Drawing for the job (mm, zero at the part's lowest x, y, z). A direction names the side the tool comes from. Round coordinates to 2 decimals unless told otherwise and drop trailing zeros. Write each loop counter-clockwise with the first axis right and the second up, starting at its lowest first coordinate (ties: lowest second). Pieces come first, ordered by that corner, then holes.
Item 1: Band-saw the part on D-D, the plane z = 5.5. Write the cut outline in (x, y), then the cut area to 3 significant figures.
Item 2: Mould opens along Z. For the marked faces 3, 4, 5 and 6 say: +Z half, -Z half, draft (parallel to the pull), parting line (faces both ways), or undercut.
Item 3: Band-saw the part on A-A, the plane y = 7.5. Write the cut outline in (x, z).
Item 4: Wall check: probe 1 along Y at (x, z) = (7.5, 4.5); probe 2 along Z at (x, y) = (4.5, 13.75); probe 3 along X at (y, z) = (6.25, 10) (1 decimal). Give the ranges that are in metal, low to high.
Item 5: 3-axis set-ups, long thin cutter, end or side, ignore diameter. For the marked faces 1 and 2: which of +Z, -Z, +X, -X, +Y, -Y reach the whole face in a straight line?
Item 6: Drop flat-ended pins along their axis: pin 1 Ø4 at (x, z) = (10, 6.5) entering from -Y; pin 2 Ø7.5 at (x, y) = (4.5, 6.5) entering from -Z; pin 3 Ø6 at (x, z) = (13, 4) entering from -Y (1 decimal); pin 4 Ø4.5 at (x, y) = (7.5, 7.5) entering from +Z. Give the stop position or say it passes through.
Item 7: Band-saw the part on C-C, the plane y = 12.25. Write the cut outline in (x, z), then the cut area to 3 significant figures.
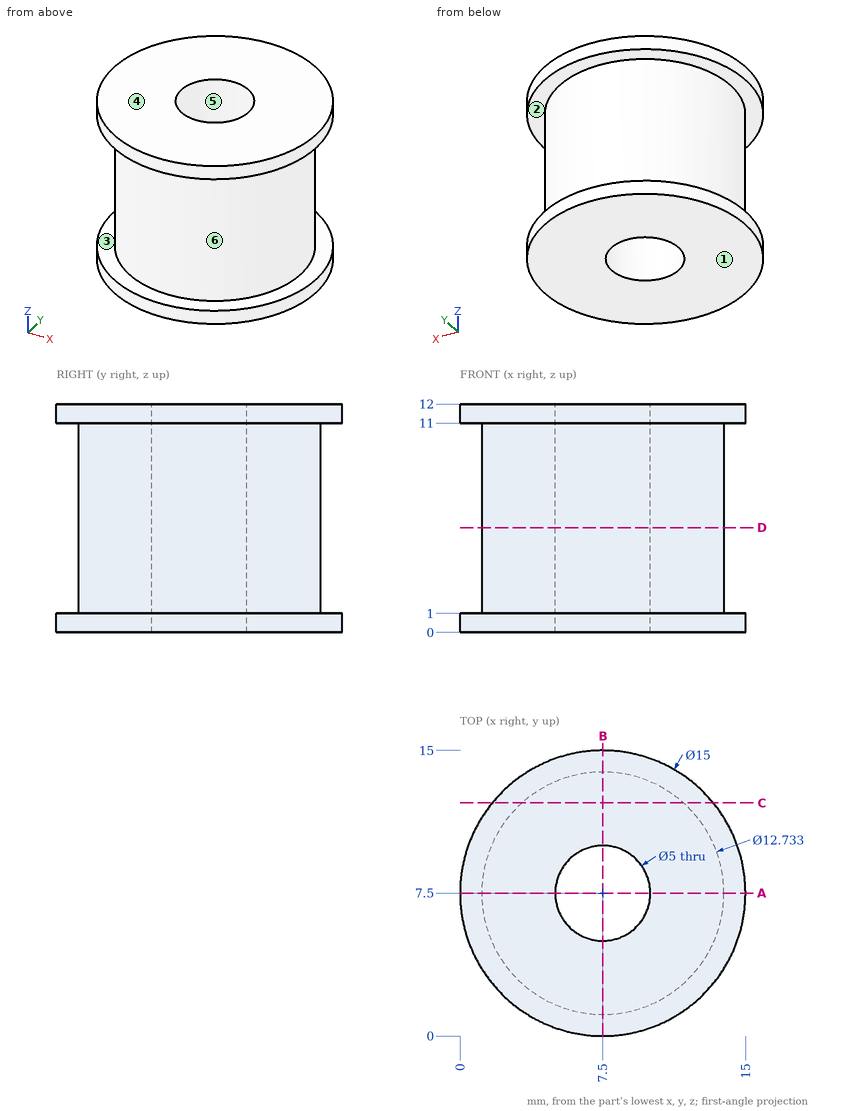
Results:
1. outline: circle Ø12.73 at (7.5, 7.5); hole circle Ø5 at (7.5, 7.5)
1. area: 108 mm2
2. face 3: undercut
2. face 4: +Z half
2. face 5: draft
2. face 6: undercut
3. outline: (0, 0) - (5, 0) - (5, 12) - (0, 12) - (0, 11) - (1.13, 11) - (1.13, 1) - (0, 1) - close; (10, 0) - (15, 0) - (15, 1) - (13.87, 1) - (13.87, 11) - (15, 11) - (15, 12) - (10, 12) - close
4. probe 1: y = 1.13 to 5, 10 to 13.87
4. probe 2: z = 0 to 1, 11 to 12
4. probe 3: x = 1.3 to 5.3, 9.7 to 13.7
5. face 1: -Z, +X, -X, +Y, -Y
5. face 2: none
6. pin 1: stops at y = 1.15
6. pin 2: stops at z = 0
6. pin 3: stops at y = 1.6
6. pin 4: passes through
7. outline: (1.7, 0) - (13.3, 0) - (13.3, 1) - (11.74, 1) - (11.74, 11) - (13.3, 11) - (13.3, 12) - (1.7, 12) - (1.7, 11) - (3.26, 11) - (3.26, 1) - (1.7, 1) - close
7. area: 108 mm2
